CAD build for the part. Positions are in the model's coordinates, mm. Coordinates: 2 decimals unless noted, no trailing zeros. Order: outer loops, then holes, each group sorted by start corner. A loop starts at its lowest first (then second) coordinate and runs counter-clockwise, first axis right, second up. Notation, with made-up numbers: (-34.75, 66) - (-20.75, 66) arc R22 ccw to (-20.75, 102) - close; hole circle Ø6 at (5, 71.5). An arc over 180 degrees is marked (long way). Use one line per item in the form item = value.
```python
from build123d import *

# Parameters (mm, degrees)
BOSS_EXTRUDE1_DEPTH            = 12.7
FILLET1_R                      = 2.54
F_97_0_31_DIAMETER_HOLE1_D     = 7.874
F_97_0_31_DIAMETER_HOLE1_DEPTH = 25.4
F_97_0_31_DIAMETER_HOLE1_TIP   = 2.365588257


with BuildPart() as part:
    # Sketch1 → Boss-Extrude1 (new body)
    with BuildSketch(Plane.XY):
        with BuildLine():
            Line((0, 12.7), (101.6, 12.7))
            ThreePointArc((101.6, 12.7), (114.3, 0), (101.6, -12.7))
            Line((101.6, -12.7), (0, -12.7))
            ThreePointArc((0, -12.7), (-12.7, 0), (0, 12.7))
        make_face()
    extrude(amount=BOSS_EXTRUDE1_DEPTH)

    # Fillet1
    fillet1_edges = [part.edges().sort_by_distance(p)[0] for p in [
        (114.3, 0, 12.7),
        (50.8, 12.7, 12.7),
        (-12.7, 0, 12.7),
        (50.8, 12.7, 0),
        (114.3, 0, 0),
        (50.8, -12.7, 0),
        (-12.7, 0, 0),
        (50.8, -12.7, 12.7),
    ]]
    fillet(fillet1_edges, radius=FILLET1_R)

    # #97 (0.31) Diameter Hole1
    with Locations(Plane.XY.offset(12.7)):
        with Locations((0, 0), (101.6, 0)):
            Hole(F_97_0_31_DIAMETER_HOLE1_D / 2, depth=F_97_0_31_DIAMETER_HOLE1_DEPTH)
            with Locations((0, 0, -(F_97_0_31_DIAMETER_HOLE1_DEPTH + F_97_0_31_DIAMETER_HOLE1_TIP / 2))):  # 118° drill point
                Cone(0, F_97_0_31_DIAMETER_HOLE1_D / 2, F_97_0_31_DIAMETER_HOLE1_TIP, mode=Mode.SUBTRACT)


solid = part.part
```
Item 1: Drop flat-ended pins along their axis: pin 1 (2 mm diameter, centred on y = 1.5, z = 7, fed in from -X); pin 2 (2 mm diameter, centred on y = -4, z = 11, fed in from -X); pin 3 (4 mm diameter, centred on y = 2.5, z = 9.5, fed in from +X). Give the stop position or say it passes through.
Derived:
pin_1 = -12.69
pin_2 = -12.28
pin_3 = 114.29
Item 2: Drill centre lines: line 1 (Y direction, x = 101.6, z = 2.75); line 2 (Y direction, x = 14.5, z = 11); line 3 (X direction, y = -10, z = 6). Where is each one in solid material? Low to high. Write a range as [from, to].
Derived:
line_1 = [-12.7, -3.94], [3.94, 12.7]
line_2 = [-12.56, 12.56]
line_3 = [-7.83, 109.43]
Item 3: Cut at B-B, the plane z = 4.25. Write the cut outline in (x, y).
Derived:
outline = (0, -12.7) - (101.6, -12.7) arc R12.7 ccw to (101.6, 12.7) - (0, 12.7) arc R12.7 ccw to start; hole circle Ø7.87 at (0, 0); hole circle Ø7.87 at (101.6, 0)
Item 4: Cut at C-C, the plane x = 30. Write the cut outline in (y, z), plus the area to 3 significant figures.
Derived:
outline = (-12.7, 2.54) arc R2.54 ccw to (-10.16, 0) - (10.16, 0) arc R2.54 ccw to (12.7, 2.54) - (12.7, 10.16) arc R2.54 ccw to (10.16, 12.7) - (-10.16, 12.7) arc R2.54 ccw to (-12.7, 10.16) - close
area = 317 mm²
Item 5: Two-plate mould, pull along X, no slides. Class faces 1 (the face through (50.089, -11.976, 0.764)), 2 (the face through (-12.697, -0.279, 6.297)), 3 (the face through (105.533, 0.173, 6.261)), 4 (the face through (0.853, -3.843, 6.261)): +X half, -X half, draft (parallel to the pull), parting line (faces both ways), or undercut.
Derived:
face_1 = draft
face_2 = -X half
face_3 = undercut
face_4 = undercut
Item 6: Cut at A-A, the plane y = 0. Write the cut outline in (x, z), plus the area to 3 significant figures.
Derived:
outline = (-12.7, 2.54) arc R2.54 ccw to (-10.16, 0) - (-3.94, 0) - (-3.94, 12.7) - (-10.16, 12.7) arc R2.54 ccw to (-12.7, 10.16) - close; (3.94, 0) - (97.66, 0) - (97.66, 12.7) - (3.94, 12.7) - close; (105.54, 0) - (111.76, 0) arc R2.54 ccw to (114.3, 2.54) - (114.3, 10.16) arc R2.54 ccw to (111.76, 12.7) - (105.54, 12.7) - close
area = 1,410 mm²
